Verification items for this drawing (mm, ordinates from the low corner). A direction names the side the tool comes from. Coordinates: 2 decimals unless noted, no trailing zeros. Write each loop counter-clockwise with the first axis right and the second up, starting at its lowest first coordinate (ties: lowest second). Pieces come first, ordered by that corner, then holes. Notation, with made-up numbers: (45, 88) -> (101, 88) arc R12 ccw to (101, 107) -> close; hole circle Ø11 at (-23.75, 6). An arc over 180 degrees is marked (long way). Use CSV: the item, a comma, the result in double quotes.
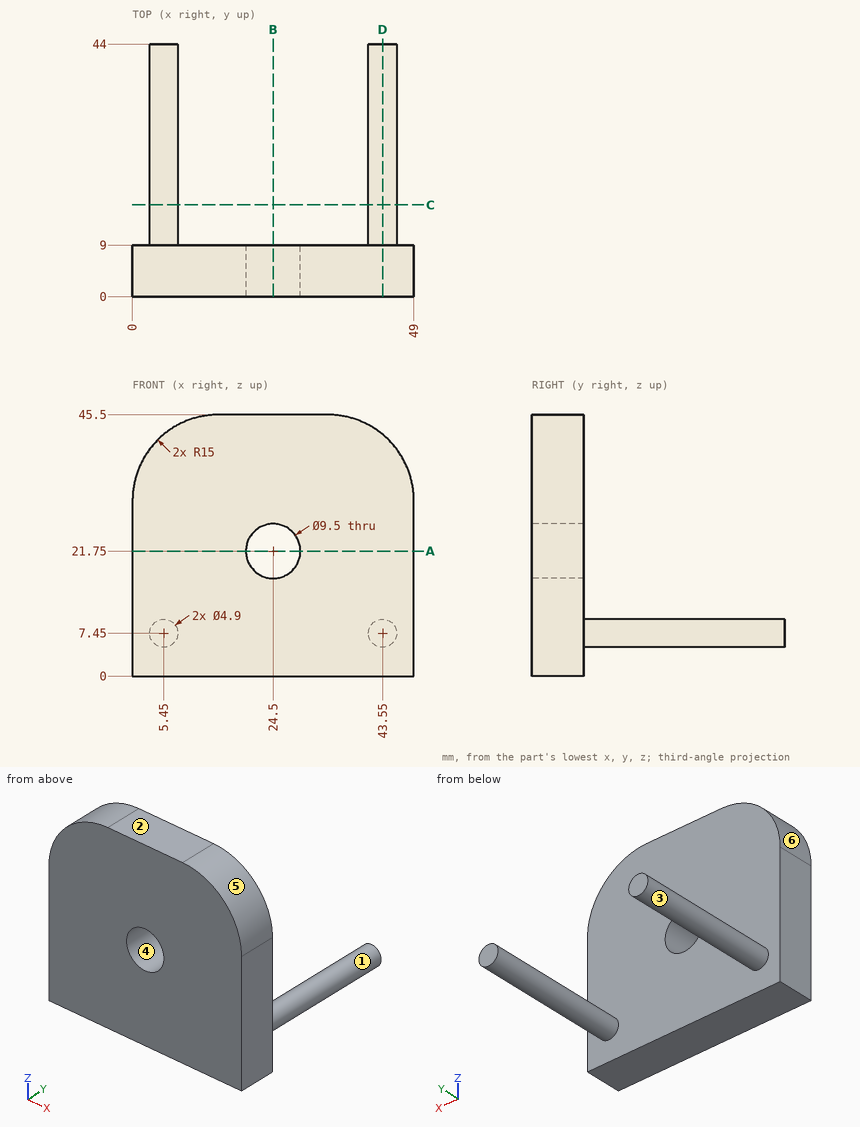
1) Set-up check for the marked faces 1 and 2: record each of +Z, -Z, +X, -X, +Y, -Y from which the full face is reachable in a straight line by a thin tool's end or side.
Return value:
face 1,"+Y"
face 2,"+Z, +X, -X, +Y, -Y"
2) Cross-section at D-D (x = 43.55). Record the boundary of the cut face in (y, z), plus the area to 3 significant figures.
Return value:
outline,"(0, 0) -> (9, 0) -> (9, 5) -> (44, 5) -> (44, 9.9) -> (9, 9.9) -> (9, 42.07) -> (0, 42.07) -> close"
area,"550 mm2"
3) Mould release check, pull along X, two halves, no side actions. Record for the marked faces 3, 4, 5 and 6: released by +X, released by -X, zero draft, split by the parting line, or undercut.
Return value:
face 3,"undercut"
face 4,"undercut"
face 5,"released by +X"
face 6,"released by -X"
4) Gauge pin test, flat ends, axial feed: pin 1 (5 mm diameter, centred on y = 20.5, z = 11, fed in from +X); pin 2 (2 mm diameter, centred on x = 38, z = 23, fed in from +Y); pin 3 (2 mm diameter, centred on x = 22, z = 23.5, fed in from +Y); pin 4 (5 mm diameter, centred on x = 8.5, y = 31, fed in from +Z). Record the tip position at first contact, or that the pin passes through.
Return value:
pin 1,"x = 45.76"
pin 2,"y = 9"
pin 3,"through"
pin 4,"z = 9.84"
5) Cross-section at B-B (x = 24.5). Record the boundary of the cut face in (y, z).
Return value:
outline,"(0, 0) -> (9, 0) -> (9, 17) -> (0, 17) -> close; (0, 26.5) -> (9, 26.5) -> (9, 45.5) -> (0, 45.5) -> close"
6) Cross-section at A-A (z = 21.75). Record the boundary of the cut face in (x, y), plus the area to 4 significant figures.
Return value:
outline,"(0, 0) -> (19.75, 0) -> (19.75, 9) -> (0, 9) -> close; (29.25, 0) -> (49, 0) -> (49, 9) -> (29.25, 9) -> close"
area,"355.5 mm2"
7) Scan lines: L1, parallel to Z at x = 24.5, y = 5; L2, parallel to Y at x = 22, z = 37; L3, parallel to X at y = 2, z = 21. Record each from-to range of solid material in increasing order.
Return value:
L1,"0 to 17, 26.5 to 45.5"
L2,"0 to 9"
L3,"0 to 19.81, 29.19 to 49"
8) Cross-section at C-C (y = 16). Record the boundary of the cut face in (x, z), plus the area to 3 significant figures.
Return value:
outline,"circle Ø4.9 at (5.45, 7.45); circle Ø4.9 at (43.55, 7.45)"
area,"37.7 mm2"
